Source: CAD feature listing. Evaluate the final solid. Frame: model axes, mm. Face numbers are marked on the shaded views. Give positions to 0.01 mm unless a question says otherwise; leave off trailing zeros. Order: outer loops, then holes, each group sorted by start corner. A loop starts at its lowest first (then second) coordinate and runs counter-clockwise, first axis right, second up. Notation, with made-up numbers: M -36,6.5 L 10,6.5 A19 ccw 10,42.5 Z; hole C 1,50.5 d1. An arc over 180 degrees is marked long. Return JSON: item names as keys, results as strings.
from build123d import *

# Parameters (mm, degrees)
F0_W        = 180
F0_H        = 116
F0_R        = 5.25
F1_DEPTH    = 20
F2_SIZE2    = 7.75
F2_SIZE     = 10
F2_2_SIZE2  = 7.75
F2_2_SIZE   = 10
F2_3_SIZE2  = 7.75
F2_3_SIZE   = 10
F2_4_SIZE2  = 7.75
F2_4_SIZE   = 10
F3_T1_DEPTH = 226.7409882636


# Not quite as in the source:
# - a fillet or chamfer that OpenCascade refuses, or shapes differently, is made with other operations: its cross-section is extruded or revolved along the edge and cut away or added


with BuildPart() as f1:
    # F0 (on Top) → F1 (new body)
    with BuildSketch(Plane.XY):
        with Locations((-6.8610161543, -3.4973233796)):
            Rectangle(F0_W, F0_H)
        with Locations((-78.8610161543, -43.4973233796)):
            Circle(F0_R, mode=Mode.SUBTRACT)
        with Locations((65.1389838457, -43.4973233796)):
            Circle(F0_R, mode=Mode.SUBTRACT)
        with Locations((-78.8610161543, 36.5026766204)):
            Circle(F0_R, mode=Mode.SUBTRACT)
        with Locations((65.1389838457, 36.5026766204)):
            Circle(F0_R, mode=Mode.SUBTRACT)
    extrude(amount=F1_DEPTH)

    # F2
    f2_edges = [f1.edges().sort_by_distance(p)[0] for p in [
        (59.888984, -43.497323, 20),
    ]]
    f2_side = f1.faces().sort_by_distance((59.888984, -43.497323, 10))[0]
    chamfer(f2_edges, length=F2_SIZE, length2=F2_SIZE2, reference=f2_side)

    # F2#2
    f2_2_edges = [f1.edges().sort_by_distance(p)[0] for p in [
        (-84.111016, -43.497323, 20),
    ]]
    f2_2_side = f1.faces().sort_by_distance((-84.111016, -43.497323, 10))[0]
    chamfer(f2_2_edges, length=F2_2_SIZE, length2=F2_2_SIZE2, reference=f2_2_side)

    # F2#3
    f2_3_edges = [f1.edges().sort_by_distance(p)[0] for p in [
        (-84.111016, 36.502677, 20),
    ]]
    f2_3_side = f1.faces().sort_by_distance((-84.111016, 36.502677, 10))[0]
    chamfer(f2_3_edges, length=F2_3_SIZE, length2=F2_3_SIZE2, reference=f2_3_side)

    # F2#4
    f2_4_edges = [f1.edges().sort_by_distance(p)[0] for p in [
        (59.888984, 36.502677, 20),
    ]]
    f2_4_side = f1.faces().sort_by_distance((59.888984, 36.502677, 10))[0]
    chamfer(f2_4_edges, length=F2_4_SIZE, length2=F2_4_SIZE2, reference=f2_4_side)

    # F3: chamfer of 9 x 2.4115427319 on 2 edges, made by hand

    # F3_s2 → F3_t1 (cut)
    with BuildSketch(Plane.YZ.offset(-120.2315102861)):
        Polygon((-52.4973233796, 20), (-61.4973233796, 17.5884572681), (-61.4973233796, 20), align=None)
        Polygon((45.5026766204, 20), (54.5026766204, 17.5884572681), (54.5026766204, 20), align=None)
    extrude(amount=F3_T1_DEPTH, mode=Mode.SUBTRACT)


solid = f1.part
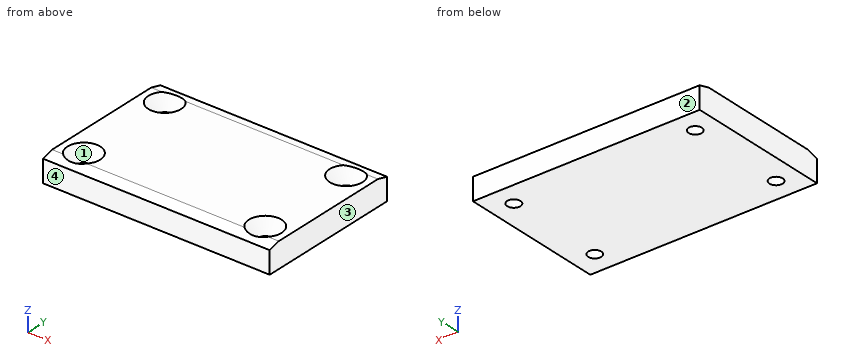
1. Section query B-B (y = -47). State how many separate pieces and enclosed holes the cut face has, then the cut area to 3 significant figures.
Evaluation:
{"separate pieces": "3", "enclosed holes": "0", "area": "3,110 mm^2"}
2. Draft query along Y for the marked faces 1, 2, 3 and 4. Return one class per face: pulls with the +Y half, pulls with the -Y half, needs draft (parallel to the pull), parting line crosses it, or undercut.
Evaluation:
{"face 1": "undercut", "face 2": "pulls with the +Y half", "face 3": "needs draft", "face 4": "pulls with the -Y half"}
3. First-contact query: pin 1 (9.5 mm diameter, centred on x = 65.14, y = -43.5, fed in from -Z) (1 decimal). Flat tip, straight axial feed; report the tip coordinate or a pass-through.
Evaluation:
{"pin 1": "passes through"}
4. Section query A-A (z = 6.25). Return loops of the section in (x, y).
Evaluation:
{"outline": "M -96.86,-61.5 L 83.14,-61.5 L 83.14,54.5 L -96.86,54.5 Z; hole C -78.86,-43.5 d10.5; hole C -78.86,36.5 d10.5; hole C 65.14,-43.5 d10.5; hole C 65.14,36.5 d10.5"}
5. Ray query, probe 1 along X at (y, z) = (-47, 18.25); probe 2 along Y at (x, z) = (68, 3.25); probe 3 along Y at (x, z) = (-78, 1.5). Return the intervals inside material, ascending.
Evaluation:
{"probe 1": "x = -96.86 to -89.97, -67.76 to 54.03, 76.24 to 83.14", "probe 2": "y = -61.5 to -47.9, -39.1 to 32.1, 40.9 to 54.5", "probe 3": "y = -61.5 to -48.68, -38.32 to 31.32, 41.68 to 54.5"}
